The drawing under review shows one solid part. Ordinate dimensions are in mm from its lowest x, y, z. Give positions to 0.01 mm unless a question says otherwise; leave off trailing zeros. Write each loop counter-clockwise with the first axis right and the second up, starting at its lowest first coordinate (ties: lowest second). Pieces come first, ordered by that corner, then holes. Notation, with made-up numbers: (20.5, -40) - (47.5, -40) arc R23 cw to (47.5, -7) - close; hole circle Ø10 at (89, 22.5). An arc over 180 degrees is marked (long way). Write item = value, one per line.
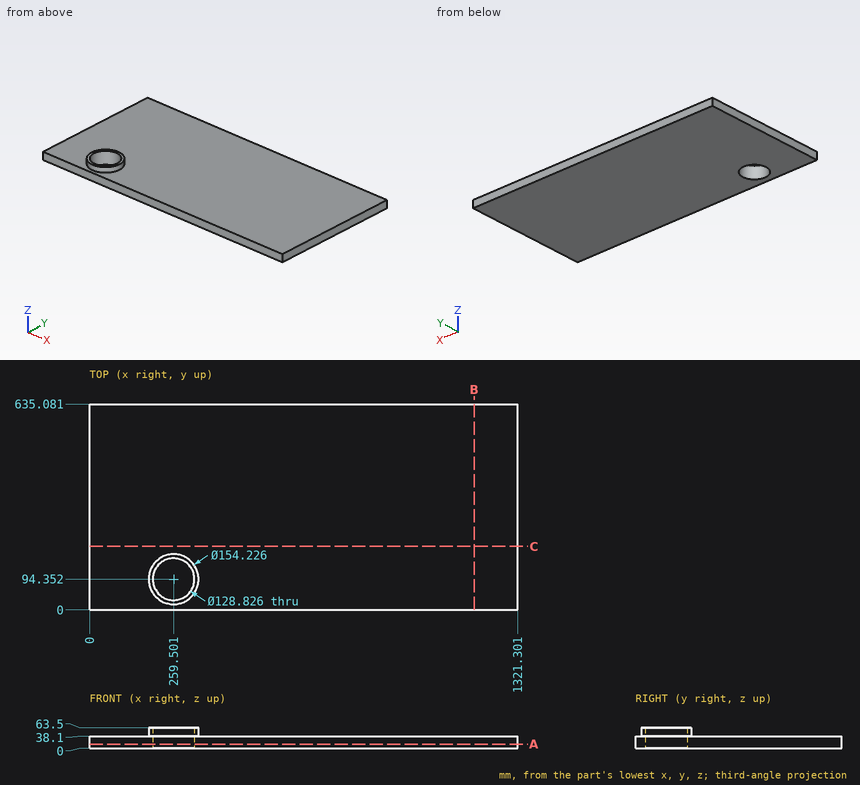
1. Insertion check: P1, Ø2, axis at x = 666, y = 559, coming from the +Z side. The pin has a flat end and moves straight along its axis. Give the tip position at first contact, or say it passes through.
Findings below:
P1 = 38.1
2. For line 1 (Z direction, x = 199, y = 434.5); line 2 (X direction, y = 103, z = 15.5); line 3 (X direction, y = 46, z = 7) (1 decimal), list the stretches that pass through material, from the lowest coordinate up. Write a range as from..to.
Findings below:
line_1 = 0..38.1
line_2 = 0..195.67, 323.33..1321.3
line_3 = 0..216.9, 302.1..1321.3
3. Take a section at A-A on z = 13. Give the boundary of the cut face in (x, y) (1 decimal), and give its area (3 significant figures).
Findings below:
outline = (0, 0) - (1321.3, 0) - (1321.3, 635.1) - (0, 635.1) - close; hole circle Ø128.8 at (259.5, 94.4)
area = 826,000 mm²
4. Take a section at B-B on x = 1186.5. Give the boundary of the cut face in (y, z), and give its area (3 significant figures).
Findings below:
outline = (0, 0) - (635.08, 0) - (635.08, 38.1) - (0, 38.1) - close
area = 24,200 mm²
5. Take a section at C-C on y = 195.5. Give the boundary of the cut face in (x, z).
Findings below:
outline = (0, 0) - (1321.3, 0) - (1321.3, 38.1) - (0, 38.1) - close
